from build123d import *

# Parameters (mm, degrees)
EXTRUDE_1_DEPTH       = 330
EXTRUDE_3_DEPTH       = 330
PATTERN_CURVE_1_DEPTH = 330
SKETCH_3_R            = 2.1
SKETCH_3_R_2          = 2.6
SKETCH_3_R_3          = 1.3
CUT_EXTRUDE_1_DEPTH   = 8
SKETCH_4_R            = 2.6
SKETCH_4_R_2          = 1.3
CUT_EXTRUDE_2_DEPTH   = 8
CUT_EXTRUDE_START     = -10
SKETCH_6_R            = 2.6
SKETCH_6_R_2          = 1.3
CUT_EXTRUDE_5_DEPTH   = 10
SKETCH_7_R            = 1.6
CUT_EXTRUDE_6_DEPTH   = 8
CUT_EXTRUDE_START_2   = -8
SKETCH_8_R            = 1.6
CUT_EXTRUDE_7_DEPTH   = 8
SKETCH_9_R            = 1.6
CUT_EXTRUDE_8_DEPTH   = 8
SKETCH_10_R           = 1.6
CUT_EXTRUDE_9_DEPTH   = 10


# Read off the part's stored shape, not the designer's step: the pattern curve step
with BuildPart() as part:
    # Sketch 1 → Extrude 1 (new body)
    with BuildSketch(Plane.XY):
        with BuildLine():
            Line((0, 45), (3.52437539, 45))
            ThreePointArc((3.52437539, 45), (3.868987923, 44.862273656), (4.02375156, 44.524968808))
            Line((4.02375156, 44.524968808), (5.5, 15))
            Line((5.5, 15), (194.5, 15))
            Line((194.5, 15), (195.97624844, 44.524968808))
            ThreePointArc((195.97624844, 44.524968808), (196.131012077, 44.862273656), (196.47562461, 45))
            Line((196.47562461, 45), (200, 45))
            Line((200, 45), (200, 0))
            Line((200, 0), (0, 0))
            Line((0, 0), (0, 45))
        make_face()
    extrude(amount=EXTRUDE_1_DEPTH)

    # Sketch 2 → Extrude 3 (add)
    with BuildSketch(Plane.XY.offset(330)):
        with BuildLine():
            Line((9.40067846, 44.428525275), (8, 15))
            Line((8, 15), (12, 15))
            Line((12, 15), (10.59932154, 44.428525275))
            ThreePointArc((10.59932154, 44.428525275), (10, 45), (9.40067846, 44.428525275))
        make_face()
    extrude(amount=-EXTRUDE_3_DEPTH)

    # Pattern Curve 1 outline → Pattern Curve 1 (add)
    with BuildSketch(Plane.XY):
        with BuildLine():
            ThreePointArc((20.59932154, 44.428525275), (20, 45), (19.40067846, 44.428525275))
            Line((19.40067846, 44.428525275), (18, 15))
            Line((18, 15), (22, 15))
            Line((22, 15), (20.59932154, 44.428525275))
        make_face()
        with BuildLine():
            Line((189.40067846, 44.428525275), (188, 15))
            Line((188, 15), (192, 15))
            Line((192, 15), (190.59932154, 44.428525275))
            ThreePointArc((190.59932154, 44.428525275), (190, 45), (189.40067846, 44.428525275))
        make_face()
        with BuildLine():
            Line((179.40067846, 44.428525275), (178, 15))
            Line((178, 15), (182, 15))
            Line((182, 15), (180.59932154, 44.428525275))
            ThreePointArc((180.59932154, 44.428525275), (180, 45), (179.40067846, 44.428525275))
        make_face()
        with BuildLine():
            Line((169.40067846, 44.428525275), (168, 15))
            Line((168, 15), (172, 15))
            Line((172, 15), (170.59932154, 44.428525275))
            ThreePointArc((170.59932154, 44.428525275), (170, 45), (169.40067846, 44.428525275))
        make_face()
        with BuildLine():
            Line((159.40067846, 44.428525275), (158, 15))
            Line((158, 15), (162, 15))
            Line((162, 15), (160.59932154, 44.428525275))
            ThreePointArc((160.59932154, 44.428525275), (160, 45), (159.40067846, 44.428525275))
        make_face()
        with BuildLine():
            Line((149.40067846, 44.428525275), (148, 15))
            Line((148, 15), (152, 15))
            Line((152, 15), (150.59932154, 44.428525275))
            ThreePointArc((150.59932154, 44.428525275), (150, 45), (149.40067846, 44.428525275))
        make_face()
        with BuildLine():
            Line((139.40067846, 44.428525275), (138, 15))
            Line((138, 15), (142, 15))
            Line((142, 15), (140.59932154, 44.428525275))
            ThreePointArc((140.59932154, 44.428525275), (140, 45), (139.40067846, 44.428525275))
        make_face()
        with BuildLine():
            Line((129.40067846, 44.428525275), (128, 15))
            Line((128, 15), (132, 15))
            Line((132, 15), (130.59932154, 44.428525275))
            ThreePointArc((130.59932154, 44.428525275), (130, 45), (129.40067846, 44.428525275))
        make_face()
        with BuildLine():
            Line((119.40067846, 44.428525275), (118, 15))
            Line((118, 15), (122, 15))
            Line((122, 15), (120.59932154, 44.428525275))
            ThreePointArc((120.59932154, 44.428525275), (120, 45), (119.40067846, 44.428525275))
        make_face()
        with BuildLine():
            Line((109.40067846, 44.428525275), (108, 15))
            Line((108, 15), (112, 15))
            Line((112, 15), (110.59932154, 44.428525275))
            ThreePointArc((110.59932154, 44.428525275), (110, 45), (109.40067846, 44.428525275))
        make_face()
        with BuildLine():
            Line((99.40067846, 44.428525275), (98, 15))
            Line((98, 15), (102, 15))
            Line((102, 15), (100.59932154, 44.428525275))
            ThreePointArc((100.59932154, 44.428525275), (100, 45), (99.40067846, 44.428525275))
        make_face()
        with BuildLine():
            Line((89.40067846, 44.428525275), (88, 15))
            Line((88, 15), (92, 15))
            Line((92, 15), (90.59932154, 44.428525275))
            ThreePointArc((90.59932154, 44.428525275), (90, 45), (89.40067846, 44.428525275))
        make_face()
        with BuildLine():
            Line((79.40067846, 44.428525275), (78, 15))
            Line((78, 15), (82, 15))
            Line((82, 15), (80.59932154, 44.428525275))
            ThreePointArc((80.59932154, 44.428525275), (80, 45), (79.40067846, 44.428525275))
        make_face()
        with BuildLine():
            Line((69.40067846, 44.428525275), (68, 15))
            Line((68, 15), (72, 15))
            Line((72, 15), (70.59932154, 44.428525275))
            ThreePointArc((70.59932154, 44.428525275), (70, 45), (69.40067846, 44.428525275))
        make_face()
        with BuildLine():
            Line((59.40067846, 44.428525275), (58, 15))
            Line((58, 15), (62, 15))
            Line((62, 15), (60.59932154, 44.428525275))
            ThreePointArc((60.59932154, 44.428525275), (60, 45), (59.40067846, 44.428525275))
        make_face()
        with BuildLine():
            Line((49.40067846, 44.428525275), (48, 15))
            Line((48, 15), (52, 15))
            Line((52, 15), (50.59932154, 44.428525275))
            ThreePointArc((50.59932154, 44.428525275), (50, 45), (49.40067846, 44.428525275))
        make_face()
        with BuildLine():
            Line((39.40067846, 44.428525275), (38, 15))
            Line((38, 15), (42, 15))
            Line((42, 15), (40.59932154, 44.428525275))
            ThreePointArc((40.59932154, 44.428525275), (40, 45), (39.40067846, 44.428525275))
        make_face()
        with BuildLine():
            Line((29.40067846, 44.428525275), (28, 15))
            Line((28, 15), (32, 15))
            Line((32, 15), (30.59932154, 44.428525275))
            ThreePointArc((30.59932154, 44.428525275), (30, 45), (29.40067846, 44.428525275))
        make_face()
    extrude(amount=PATTERN_CURVE_1_DEPTH)

    # Sketch 3 → Cut-Extrude 1 (cut)
    with BuildSketch(Plane.XZ):
        with Locations((9.5, 19.5)):
            Circle(SKETCH_3_R)
        with Locations((188.5, 40)):
            Circle(SKETCH_3_R)
        with Locations((163.5, 130)):
            Circle(SKETCH_3_R)
        with Locations((11.5, 151)):
            Circle(SKETCH_3_R)
        with Locations((63.5, 189)):
            Circle(SKETCH_3_R)
        with Locations((16.5, 240)):
            Circle(SKETCH_3_R)
        with Locations((39.5, 79.5)):
            Circle(SKETCH_3_R_2)
        with Locations((114.5, 30)):
            Circle(SKETCH_3_R)
        with Locations((181.5, 210)):
            Circle(SKETCH_3_R)
        with Locations((16.58, 183.75)):
            Circle(SKETCH_3_R_2)
        with Locations((84, 49)):
            Circle(SKETCH_3_R_3)
        with Locations((89, 89)):
            Circle(SKETCH_3_R_3)
        with Locations((61.5, 170)):
            Circle(SKETCH_3_R_3)
        with Locations((61.5, 210)):
            Circle(SKETCH_3_R_3)
        with Locations((108.5, 190)):
            Circle(SKETCH_3_R_3)
        with Locations((138, 189.5)):
            Circle(SKETCH_3_R)
    extrude(amount=-CUT_EXTRUDE_1_DEPTH, mode=Mode.SUBTRACT)

    # Sketch 4 → Cut-Extrude 2 (cut)
    with BuildSketch(Plane.ZY):
        with Locations(Location((30, 15, 0), (0, 0, 270))):
            Circle(SKETCH_4_R)
        with Locations(Location((75, 15, 0), (0, 0, 270))):
            Circle(SKETCH_4_R_2)
        with Locations(Location((120, 15, 0), (0, 0, 270))):
            Circle(SKETCH_4_R)
        with Locations((210, 15)):
            Circle(SKETCH_4_R)
        with Locations((255, 15)):
            Circle(SKETCH_4_R_2)
        with Locations((300, 15)):
            Circle(SKETCH_4_R)
    extrude(amount=-CUT_EXTRUDE_2_DEPTH, mode=Mode.SUBTRACT)

    # Sketch 6 → Cut-Extrude 5 (cut)
    with BuildSketch(Plane(origin=(200, 0, 0), x_dir=(0, 0, -1), z_dir=(1, 0, 0)).offset(CUT_EXTRUDE_START)):
        with Locations(Location((-30, 15, 0), (0, 0, 270))):
            Circle(SKETCH_6_R)
        with Locations(Location((-75, 15, 0), (0, 0, 270))):
            Circle(SKETCH_6_R_2)
        with Locations(Location((-120, 15, 0), (0, 0, 270))):
            Circle(SKETCH_6_R)
        with Locations(Location((-210, 15, 0), (0, 0, 180))):
            Circle(SKETCH_6_R)
        with Locations(Location((-255, 15, 0), (0, 0, 180))):
            Circle(SKETCH_6_R_2)
        with Locations(Location((-300, 15, 0), (0, 0, 180))):
            Circle(SKETCH_6_R)
    extrude(amount=CUT_EXTRUDE_5_DEPTH, mode=Mode.SUBTRACT)

    # Sketch 7 → Cut-Extrude 6 (cut)
    with BuildSketch(Plane.XY.offset(330)):
        with Locations((30, 7.5)):
            Circle(SKETCH_7_R)
        with Locations((170, 7.5)):
            Circle(SKETCH_7_R)
    extrude(amount=-CUT_EXTRUDE_6_DEPTH, mode=Mode.SUBTRACT)

    # Sketch 8 → Cut-Extrude 7 (cut)
    with BuildSketch(Plane(origin=(0, 0, 0), x_dir=(-1, 0, 0), z_dir=(0, 0, -1)).offset(CUT_EXTRUDE_START_2)):
        with Locations(Location((-30, 7.5, 0), (0, 0, 180))):
            Circle(SKETCH_8_R)
        with Locations(Location((-170, 7.5, 0), (0, 0, 180))):
            Circle(SKETCH_8_R)
    extrude(amount=CUT_EXTRUDE_7_DEPTH, mode=Mode.SUBTRACT)

    # Sketch 9 → Cut-Extrude 8 (cut)
    with BuildSketch(Plane.XZ):
        with Locations((147, 320)):
            Circle(SKETCH_9_R)
        with Locations((147, 265)):
            Circle(SKETCH_9_R)
    extrude(amount=-CUT_EXTRUDE_8_DEPTH, mode=Mode.SUBTRACT)

    # Sketch 10 → Cut-Extrude 9 (cut)
    with BuildSketch(Plane.XZ):
        with Locations((111.453923093, 292.5)):
            Circle(SKETCH_10_R)
        with Locations((182.546076907, 292.5)):
            Circle(SKETCH_10_R)
    extrude(amount=-CUT_EXTRUDE_9_DEPTH, mode=Mode.SUBTRACT)


solid = part.part
Can you work these out from the model? Positions are in its coordinate system, mm. Give positions to 0.01 mm unless a question says otherwise; leave off trailing zeros. Return JSON: item names as keys, results as strings.
1. I'm going to push flat-ended pins straight in: pin 1 Ø2.5 at (x, y) = (30, 7.5) entering from -Z; pin 2 Ø1.8 at (x, z) = (46, 240) entering from +Y; pin 3 Ø2.5 at (x, z) = (147, 265) entering from -Y. Where does each tip first touch, or does it pass through?
Output values:
{"pin 1": "stops at z = 8", "pin 2": "stops at y = 15", "pin 3": "stops at y = 8"}
2. If I drill on line 1 (Z direction, x = 147, y = 2.75); line 2 (Y direction, x = 30, z = 324.5); line 3 (X direction, y = 6, z = 40.5), over which ranges is the centre line in solid material (lowest first)?
Output values:
{"line 1": "z = 0 to 263.4, 266.6 to 318.4, 321.6 to 330", "line 2": "y = 0 to 5.9, 9.1 to 45", "line 3": "x = 0 to 186.46, 190.54 to 200"}
3. I want a section at A-A on y = 28. Give the number of separate pieces and of enclosed holes in the cut face, and give its area (3 significant figures).
Output values:
{"separate pieces": "21", "enclosed holes": "0", "area": "20,500 mm²"}
